The listing builds one solid part. Answer for the finished solid, in the listing's coordinates (mm). Face numbers are marked on the shaded views. A direction names the side the tool comes from. Round coordinates to 2 decimals unless told otherwise and drop trailing zeros. Loops run counter-clockwise (first coordinate to the right, second up) from the corner with the lowest first, then second, coordinate; pieces in that order, holes last. Notation, with made-up numbers: (-37, 76.25) - (-8, 76.25) arc R13 cw to (-8, 100.25) - close; hole circle Ø2 at (-1, -22). An arc over 180 degrees is marked (long way). One line per item, written item: value.
```python
from build123d import *

# Parameters (mm, degrees)
F0_R          = 3.175
F0_W          = 5.842
F0_H          = 12.7
F2_DEPTH      = 3.175
F2_DEPTH_BACK = 3.175
F3_R          = 1.524
F4_DEPTH      = 6.35
F4_DEPTH_BACK = 1.27
F5_DEPTH      = 56.134
F8_DEPTH      = 17.78
F9_DEPTH      = 10.414


with BuildPart() as f1:
    # F0 (on Front) → F1 (revolve)
    with BuildSketch(Plane.XZ):
        Polygon((5.842, 12.7), (5.842, 0), (66.294, 0), (66.294, 12.7), (56.134, 12.7), (56.134, 10.16), (10.16, 10.16), (10.16, 12.7), align=None)
    revolve(axis=Axis((-3.3274, 0, 0), (-1, 0, 0)))

    # F0 (on Front) → F2 (join, two sides)
    with BuildSketch(Plane.XZ) as f2_sk:
        with BuildLine():
            Line((5.842, 0), (0, 0))
            Line((0, 0), (-0.9398, 0))
            ThreePointArc((-0.9398, 0), (-3.1957909266, -4.5493385486), (-8.1826630726, -5.5069827884))
            Line((-8.1826630726, -5.5069827884), (5.842, -9.398))
            Line((5.842, -9.398), (5.842, 0))
        make_face()
        with BuildLine():
            Line((-0.9398, 0), (0, 0))
            Line((0, 0), (0, 12.7))
            Line((0, 12.7), (5.842, 12.7))
            Line((5.842, 12.7), (5.842, 15.24))
            Line((5.842, 15.24), (-0.508, 15.24))
            Line((-0.508, 15.24), (-10.8806298187, 3.8475430269))
            ThreePointArc((-10.8806298187, 3.8475430269), (-4.5919612295, 5.3297205562), (-0.9398, 0))
        make_face()
        with BuildLine():
            ThreePointArc((-8.1826630726, -5.5069827884), (-3.1957909266, -4.5493385486), (-0.9398, 0))
            ThreePointArc((-0.9398, 0), (-4.5919612295, 5.3297205562), (-10.8806298187, 3.8475430269))
            ThreePointArc((-10.8806298187, 3.8475430269), (-12.1459778134, -1.5837270034), (-8.1826630726, -5.5069827884))
        make_face()
        with Locations((-6.6548, 0)):
            Circle(F0_R, mode=Mode.SUBTRACT)
        with Locations((2.921, 6.35)):
            Rectangle(F0_W, F0_H)
    extrude(amount=F2_DEPTH)
    extrude(f2_sk.sketch, amount=-F2_DEPTH_BACK)

    # F3 (on face) → F4 (join, two sides)
    with BuildSketch(Plane.YZ.offset(66.294)) as f4_sk:
        with BuildLine():
            ThreePointArc((-5.08, 11.6397422652), (-0.0019395312, 12.6999998519), (5.0764445437, 11.6412933472))
            Line((5.0764445437, 11.6412933472), (5.0753448882, 15.241550914))
            Line((5.0753448882, 15.241550914), (-0.0176815379, 15.241550914))
            Line((-0.0176815379, 15.241550914), (-5.08, 15.241550914))
            Line((-5.08, 15.241550914), (-5.08, 11.6397422652))
        make_face()
        with BuildLine():
            ThreePointArc((-5.08, 0), (-0.0007758125, 5.0799999408), (5.079999763, 0.0015516249))
            Line((5.079999763, 0.0015516249), (5.0764445437, 11.6412933472))
            ThreePointArc((5.0764445437, 11.6412933472), (-0.0019395312, 12.6999998519), (-5.08, 11.6397422652))
            Line((-5.08, 11.6397422652), (-5.08, 0))
        make_face()
        with BuildLine():
            ThreePointArc((-5.08, 0), (0, -5.08), (5.08, 0))
            ThreePointArc((5.08, 0), (5.0799999408, 0.0007758125), (5.079999763, 0.0015516249))
            ThreePointArc((5.079999763, 0.0015516249), (-0.0007758125, 5.0799999408), (-5.08, 0))
        make_face()
        Circle(F3_R, mode=Mode.SUBTRACT)
    extrude(amount=F4_DEPTH)
    extrude(f4_sk.sketch, amount=-F4_DEPTH_BACK)

    # F5 (cut, through all): a face of the model
    f5_faces = [f1.faces().sort_by_distance(p)[0] for p in [
        (66.294, 0, 0),
    ]]
    extrude(f5_faces, amount=-F5_DEPTH, mode=Mode.SUBTRACT)

    # F6 (on face) → F8 (cut)
    with BuildSketch(Plane.XY.offset(15.24)):
        with BuildLine():
            ThreePointArc((2.667, -1.524), (3.7446307345, -1.0776307345), (4.191, 0))
            ThreePointArc((4.191, 0), (3.7446307345, 1.0776307345), (2.667, 1.524))
            Line((2.667, 1.524), (2.667, 0))
            Line((2.667, 0), (2.667, -1.524))
        make_face()
        with BuildLine():
            Line((2.667, 0), (2.667, 1.524))
            ThreePointArc((2.667, 1.524), (1.143, 0), (2.667, -1.524))
            Line((2.667, -1.524), (2.667, 0))
        make_face()
    extrude(amount=-F8_DEPTH, mode=Mode.SUBTRACT)

    # F7 (on face) → F9 (cut)
    with BuildSketch(Plane.XY.offset(15.241550914)):
        with BuildLine():
            Line((68.834, -0.0023275559), (68.834, 1.5216724441))
            ThreePointArc((68.834, 1.5216724441), (67.7563692655, 1.0753031786), (67.31, -0.0023275559))
            Line((67.31, -0.0023275559), (68.834, -0.0023275559))
        make_face()
        with BuildLine():
            ThreePointArc((70.358, -0.0023275559), (69.9116307345, 1.0753031786), (68.834, 1.5216724441))
            Line((68.834, 1.5216724441), (68.834, -0.0023275559))
            Line((68.834, -0.0023275559), (70.358, -0.0023275559))
        make_face()
        with BuildLine():
            Line((68.834, -1.5263275559), (68.834, -0.0023275559))
            Line((68.834, -0.0023275559), (67.31, -0.0023275559))
            ThreePointArc((67.31, -0.0023275559), (67.7563692655, -1.0799582904), (68.834, -1.5263275559))
        make_face()
        with BuildLine():
            Line((70.358, -0.0023275559), (68.834, -0.0023275559))
            Line((68.834, -0.0023275559), (68.834, -1.5263275559))
            ThreePointArc((68.834, -1.5263275559), (69.9116307345, -1.0799582904), (70.358, -0.0023275559))
        make_face()
    extrude(amount=-F9_DEPTH, mode=Mode.SUBTRACT)


solid = f1.part
```
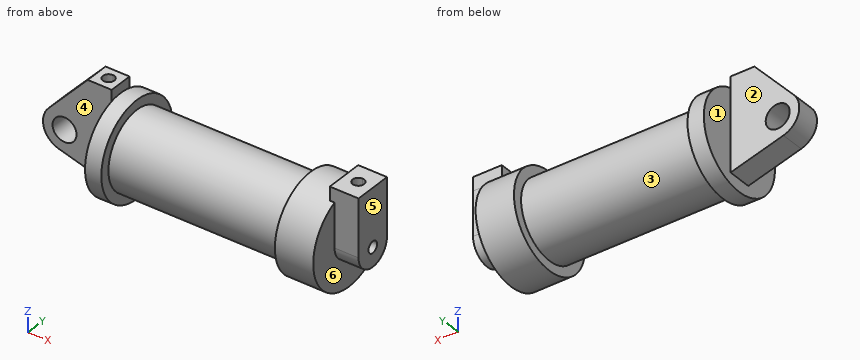
1) A cutting plane is placed at A-A on z = -0.75. Give the number of separate pieces and of enclosed holes in the cut face, and give its area (3 significant figures).
Final values:
separate pieces: 2
enclosed holes: 1
area: 1,270 mm2
2) A cutting plane is placed at C-C on y = 4. Give the vertices of the cut face in (x, z), and give its area (3 significant figures).
Final values:
outline: (5.84, -12.05) - (10.16, -12.05) - (10.16, -9.34) - (56.13, -9.34) - (56.13, -12.05) - (66.29, -12.05) - (66.29, -3.13) - (72.64, -3.13) - (72.64, 15.24) - (65.02, 15.24) - (65.02, 12.05) - (56.13, 12.05) - (56.13, 9.34) - (10.16, 9.34) - (10.16, 12.05) - (5.84, 12.05) - close
area: 1,330 mm2
3) For a pull along X with two mould halves and no side action, classify the marked faces 1, 2 and 3 as released by +X, released by -X, zero draft, split by the parting line, or undercut.
Final values:
face 1: released by -X
face 2: zero draft
face 3: undercut
4) Consider L1, parallel to X at y = -10, z = 4.75; L2, parallel to Y at x = 2.5, z = 5 (3 decimals); L3, parallel to X at y = 2.25, z = 1.25. Determine where each line is inside the solid, lowest interval first.
Final values:
L1: 5.84 to 10.16, 56.13 to 66.29
L2: -3.175 to -1.515, 1.515 to 3.175
L3: -12.23 to -9.57, -3.74 to 72.64
5) Each of these flat-tipped pins is pushed along its axis until it touches: pin 1 Ø7.5 at (y, z) = (-5, -4.5) entering from -X; pin 2 Ø1.5 at (x, z) = (62, -6.5) entering from +Y; pin 3 Ø0.9 at (x, y) = (2.5, -0.5) entering from +Z; pin 4 Ø2 at (x, z) = (11.5, 12.5) entering from -Y. Where does it stop, or does it pass through?
Final values:
pin 1: x = -12.24
pin 2: y = 11.32
pin 3: z = -2.54
pin 4: through
6) A cutting plane is placed at B-B on x = 12. Give the vertices of the cut face in (y, z), and give its area (3 significant figures).
Final values:
outline: circle Ø20.32 at (0, 0); hole circle Ø3.05 at (0, 0)
area: 317 mm2
7) A cutting plane is placed at D-D on z = 7. Give the vertices of the cut face in (x, y) (3 decimals), and give its area (3 significant figures).
Final values:
outline: (-8.01, -3.175) - (5.842, -3.175) - (5.842, -10.597) - (10.16, -10.597) - (10.16, -7.364) - (56.134, -7.364) - (56.134, -10.597) - (66.294, -10.597) - (66.294, -5.08) - (72.644, -5.08) - (72.644, 5.078) - (66.294, 5.078) - (66.294, 10.597) - (56.134, 10.597) - (56.134, 7.364) - (10.16, 7.364) - (10.16, 10.597) - (5.842, 10.597) - (5.842, 3.175) - (-8.01, 3.175) - close; hole circle Ø3.048 at (2.667, 0); hole circle Ø3.048 at (68.834, -0.002)
area: 1,120 mm2
8) For the marked faces 4, 5 and 6, determine the directions among +Z, -Z, +X, -X, +Y, -Y from which every point of the face is accessible in a straight line to the end or side of a thin tool.
Final values:
face 4: +Z, -Z, -X, -Y
face 5: +Z, -Z, +X, +Y, -Y
face 6: -Z, +X
